Read the model definition and answer for the solid it produces. Units are mm, in the model's axes. Face numbers are marked on the shaded views. A direction names the side the tool comes from. Coordinates: 2 decimals unless noted, no trailing zeros. Write each loop counter-clockwise with the first axis right and the second up, starting at its lowest first coordinate (ties: lowest second). Pieces come first, ordered by that corner, then holes. Notation, with made-up numbers: (12, -28.75) -> (66, -28.75) arc R32 cw to (66, -2.75) -> close; hole circle Ø1 at (-21.5, -4). An arc over 180 degrees is marked (long way). Return JSON: item names as keys, results as strings.
from build123d import *

# Parameters (mm, degrees)
SKETCH1_RX          = 70
SKETCH1_RY          = 30
BOSS_EXTRUDE1_DEPTH = 30


with BuildPart() as part:
    # Sketch1 → Boss-Extrude1 (new body)
    with BuildSketch(Plane.XY):
        with BuildLine():
            Line((130, -70), (70, -70))
            Line((70, -70), (70, -40))
            Line((70, -40), (40, -40))
            Line((40, -40), (40, -70))
            Line((40, -70), (-40, -70))
            Line((-40, -70), (-40, -40))
            Line((-40, -40), (-70, -40))
            Line((-70, -40), (-70, -70))
            Line((-70, -70), (-130, -70))
            Line((-130, -70), (-130, 70))
            Line((-130, 70), (-80, 70))
            Line((-80, 70), (-80, 100))
            ThreePointArc((-80, 100), (0, 180), (80, 100))
            Line((80, 100), (80, 70))
            Line((80, 70), (130, 70))
            Line((130, 70), (130, -70))
        make_face()
        with Locations(Location((0, 28.005273926), (0, 0, -180))):
            Ellipse(SKETCH1_RX, SKETCH1_RY, mode=Mode.SUBTRACT)
        with BuildLine():
            ThreePointArc((66, 100), (0, 166), (-66, 100))
            ThreePointArc((-66, 100), (-55, 89), (-44, 100))
            ThreePointArc((-44, 100), (0, 144), (44, 100))
            ThreePointArc((44, 100), (55, 89), (66, 100))
        make_face(mode=Mode.SUBTRACT)
    extrude(amount=BOSS_EXTRUDE1_DEPTH)


solid = part.part
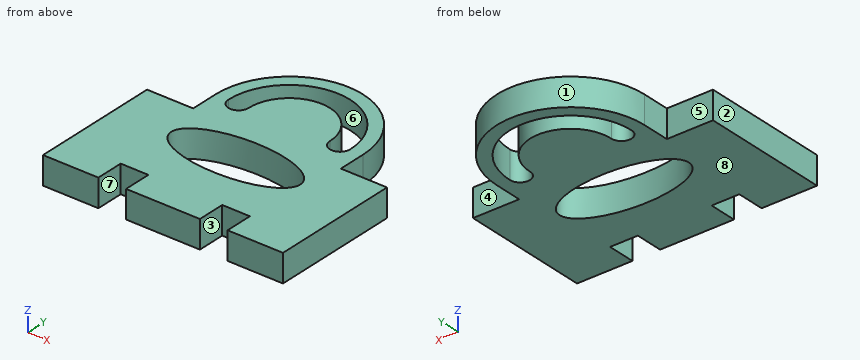
1. The part is cut by section D-D (x = 103). Determine the outline of the cut face in (y, z).
Taken from the geometry:
{"outline": "(-70, 0) -> (70, 0) -> (70, 30) -> (-70, 30) -> close"}
2. Flat-ended cylindrical pins translate along their axes: pin 1 Ø8 at (y, z) = (151.5, 25) entering from -X; pin 2 Ø8 at (x, y) = (-58, 52.5) entering from -Z; pin 3 Ø3 at (x, z) = (48, 16.5) entering from -Y; pin 4 Ø15 at (x, z) = (-96, 21) entering from +Y. Find the tip coordinate at first contact, or state that the pin passes through.
Taken from the geometry:
{"pin 1": "stops at x = -64.37", "pin 2": "stops at z = 0", "pin 3": "stops at y = -40", "pin 4": "stops at y = 70"}
3. For a pull along X with two mould halves and no side action, classify the marked faces 1, 2 and 3 as +X half, -X half, draft (parallel to the pull), parting line (faces both ways), or undercut.
Taken from the geometry:
{"face 1": "parting line", "face 2": "-X half", "face 3": "undercut"}
4. Consider L1, parallel to Y at x = -35.5, z = 21.75; L2, parallel to Y at x = 48.5, z = 23.5; L3, parallel to X at y = 121, z = 27.5. Determine where each line is inside the solid, lowest interval first.
Taken from the geometry:
{"L1": "y = -70 to 2.15, 53.86 to 126, 155.64 to 171.69", "L2": "y = -40 to 6.37, 49.64 to 91.13, 144.76 to 163.62", "L3": "x = -77.19 to -62.57, -38.67 to 38.67, 62.57 to 77.19"}
5. The part is cut by section B-B (x = 0). Count the separate pieces of the cut face and the enclosed holes in it, then the cut area to 3 significant figures.
Taken from the geometry:
{"separate pieces": "3", "enclosed holes": "0", "area": "5,040 mm2"}
6. A tool of negligible diameter and unlimited length cuts with its end or side. For the marked faces 4, 5, 6, 7 and 8, from which of +Z, -Z, +X, -X, +Y, -Y can it reach the whole face along a straight path? Write none if from no direction.
Taken from the geometry:
{"face 4": "+Z, -Z, +X, +Y", "face 5": "+Z, -Z, -X, +Y", "face 6": "+Z, -Z", "face 7": "+Z, -Z, -Y", "face 8": "-Z, +X, -X, +Y, -Y"}
7. The part is cut by section A-A (y = -52.5). Determine the outline of the cut face in (x, z), then the cut area to 3 significant figures.
Taken from the geometry:
{"outline": "(-130, 0) -> (-70, 0) -> (-70, 30) -> (-130, 30) -> close; (-40, 0) -> (40, 0) -> (40, 30) -> (-40, 30) -> close; (70, 0) -> (130, 0) -> (130, 30) -> (70, 30) -> close", "area": "6,000 mm2"}
